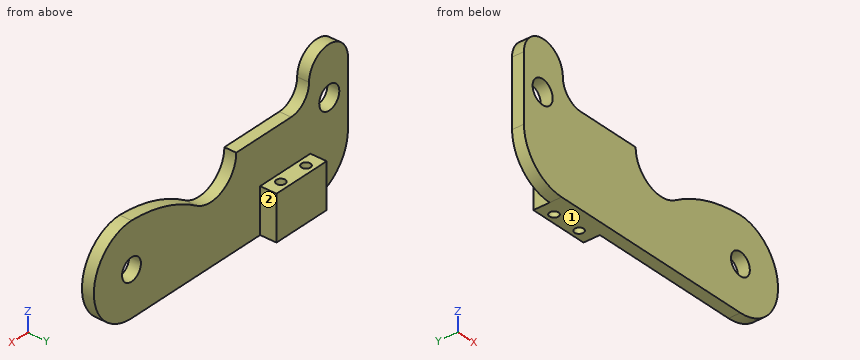
```python
from build123d import *

# Parameters (mm, degrees)
SKETCH1_R           = 1.5
SKETCH1_R_2         = 1.6
BOSS_EXTRUDE1_DEPTH = 1.6
SKETCH2_W           = 8
SKETCH2_H           = 6
BOSS_EXTRUDE2_DEPTH = 2.2
CUT_EXTRUDE1_REACH  = 77.825
SKETCH3_R           = 0.6
FILLET1_R           = 20


with BuildPart() as part:
    # Sketch1 → Boss-Extrude1 (new body)
    with BuildSketch(Plane(origin=(0, 0, 0), x_dir=(1, 0, 0), z_dir=(0, 1, 0))):
        with BuildLine():
            Line((33.072085441, -182.752493772), (33.072085441, -191.652493772))
            ThreePointArc((33.072085441, -191.652493772), (36.172085441, -194.752493772), (39.272085441, -191.652493772))
            ThreePointArc((39.272085441, -191.652493772), (40.106831114, -189.637239445), (42.122085441, -188.802493772))
            Line((42.122085441, -188.802493772), (50.872085441, -188.802493772))
            ThreePointArc((50.872085441, -188.802493772), (54.922085441, -184.752493772), (58.972085441, -188.802493772))
            Line((58.972085441, -188.802493772), (67.571877104, -188.802493772))
            ThreePointArc((67.571877104, -188.802493772), (73.571877104, -182.802493772), (67.571877104, -176.802493772))
            Line((67.571877104, -176.802493772), (39.071877104, -176.802493772))
            ThreePointArc((39.071877104, -176.802493772), (34.846951069, -178.542212091), (33.072085441, -182.752493772))
        make_face()
        with Locations(Location((67.571877104, -182.802493772, 0), (0, 0, 270))):
            Circle(SKETCH1_R, mode=Mode.SUBTRACT)
        with Locations(Location((36.052926365, -188.193770201, 0), (0, 0, 270))):
            Circle(SKETCH1_R_2, mode=Mode.SUBTRACT)
    extrude(amount=BOSS_EXTRUDE1_DEPTH)

    # Sketch2 → Boss-Extrude2 (add)
    with BuildSketch(Plane(origin=(0, 1.6, 0), x_dir=(1, 0, 0), z_dir=(0, 1, 0))):
        with Locations((43.071877104, -179.802493772)):
            Rectangle(SKETCH2_W, SKETCH2_H)
    extrude(amount=BOSS_EXTRUDE2_DEPTH)

    # Sketch3 → Cut-Extrude1 (cut, up to next)
    with BuildSketch(Plane(origin=(0, 0, 176.802493772), x_dir=(-1, 0, 0), z_dir=(0, 0, -1)), mode=Mode.PRIVATE) as cut_extrude1_sk1:
        with Locations((-45.071877104, 2.7)):
            Circle(SKETCH3_R)
    cut_extrude1_tool1 = extrude(cut_extrude1_sk1.sketch, amount=-CUT_EXTRUDE1_REACH, mode=Mode.PRIVATE) & part.part
    # Sketch3 → Cut-Extrude1 (cut, up to next)
    with BuildSketch(Plane(origin=(0, 0, 176.802493772), x_dir=(-1, 0, 0), z_dir=(0, 0, -1)), mode=Mode.PRIVATE) as cut_extrude1_sk2:
        with Locations((-41.071877104, 2.7)):
            Circle(SKETCH3_R)
    cut_extrude1_tool2 = extrude(cut_extrude1_sk2.sketch, amount=-CUT_EXTRUDE1_REACH, mode=Mode.PRIVATE) & part.part
    add(cut_extrude1_tool1.solids().sort_by_distance((45.071877, 2.7, 176.802494))[0], mode=Mode.SUBTRACT)
    add(cut_extrude1_tool2.solids().sort_by_distance((41.071877, 2.7, 176.802494))[0], mode=Mode.SUBTRACT)

    # Fillet1
    # the kernel refuses this fillet: 20 mm, written as the material it takes off along each edge
    with BuildSketch(Plane(origin=(58.972085441, -21.499479158, 188.802493772), x_dir=(-0.47106518434260986, 0, -0.8820984027308195), z_dir=(0, 1, 0))) as fillet1_piece_1:
        with BuildLine():
            CenterArc((13.23693168, -17.641968055), FILLET1_R, 118.103462193, 31.710767892)
            Line((-4.051062445, -7.58586249), (0, 0))
            ThreePointArc((0, 0), (1.907813997, -0.477501469), (3.815627993, 0))
        make_face()
    extrude(amount=44.598958315, mode=Mode.SUBTRACT)


solid = part.part
```
Model file for the job. Use its own axes, mm. Face numbers are marked on the shaded views. A direction names the side the tool comes from. Give positions to 0.01 mm unless a question says otherwise; leave off trailing zeros. Loops run counter-clockwise (first coordinate to the right, second up) from the corner with the lowest first, then second, coordinate; pieces in that order, holes last. Notation, with made-up numbers: M 70,13.5 L 91,13.5 A12 cw 91,18.5 Z; hole C 86,52.25 d2. An arc over 180 degrees is marked long. Use one line per item in the form item = value.
Item 1: Flat gauge pins, fed straight in: pin 1 Ø6 at (x, z) = (62, 181) entering from -Y; pin 2 Ø1.8 at (x, y) = (44.5, 3) entering from +Z; pin 3 Ø4 at (x, z) = (36.05, 188.19) entering from +Y; pin 4 Ø1.5 at (y, z) = (1, 184.5) entering from +X. Where does each tip first touch, or does it go through?
Filled in:
pin_1 = 0
pin_2 = 182.8
pin_3 = 1.6
pin_4 = 73.5
Item 2: Slice it at A-A on y = 2.7. List the corners of the cut face in (x, z).
Filled in:
outline = M 39.07,176.8 L 40.47,176.8 L 40.47,182.8 L 39.07,182.8 Z; M 41.67,176.8 L 44.47,176.8 L 44.47,182.8 L 41.67,182.8 Z; M 45.67,176.8 L 47.07,176.8 L 47.07,182.8 L 45.67,182.8 Z
Item 3: Which spindle directions (+Z, -Z, +X, -X, +Y, -Y) get a long thin tool onto all of the face, cutting with end or side? Do the marked faces 1 and 2. Say none if no direction does.
Filled in:
face_1 = -Z, +X, -X, +Y, -Y
face_2 = +Z, -Z, +X, +Y
Item 4: Slice it at B-B on z = 187. List the corners of the cut face in (x, y), and give its area (3 significant figures).
Filled in:
outline = M 33.07,0 L 34.99,0 L 34.99,1.6 L 33.07,1.6 Z; M 37.12,0 L 51.3,0 L 51.3,1.6 L 37.12,1.6 Z; M 59.97,0 L 71.86,0 L 71.86,1.6 L 59.97,1.6 Z
area = 44.8 mm^2
Item 5: Drill centre lines: L1, parallel to X at y = 3.1, z = 182.25; L2, parallel to Y at x = 64, z = 180; L3, parallel to X at y = 3.2, z = 180.25. Where is each one in solid material? Low to high.
Filled in:
L1 = 39.07 to 40.62, 41.52 to 44.62, 45.52 to 47.07
L2 = 0 to 1.6
L3 = 39.07 to 40.74, 41.4 to 44.74, 45.4 to 47.07
Item 6: Slice it at C-C on x = 43. List the corners of the cut face in (y, z), and give its area (3 significant figures).
Filled in:
outline = M 0,176.8 L 3.8,176.8 L 3.8,182.8 L 1.6,182.8 L 1.6,188.8 L 0,188.8 Z
area = 32.4 mm^2
Item 7: Slice it at D-D on x = 59.5. List the corners of the cut face in (y, z), and give its area (3 significant figures).
Filled in:
outline = M 0,176.8 L 1.6,176.8 L 1.6,186.78 L 0,186.78 Z
area = 16.0 mm^2
